Verification items for the finished model (mm, model axes). A direction names the side the tool comes from. Round coordinates to 2 decimals unless told otherwise and drop trailing zeros. Write each loop counter-clockwise with the first axis right and the second up, starting at its lowest first coordinate (ties: lowest second). Pieces come first, ordered by that corner, then holes. Notation, with made-up numbers: M -27.75,-32 L 7.25,-32 A15 ccw 7.25,-9 Z; hole C -29,80.25 d5. An arc over 180 degrees is marked long. Write each question's results on one line, items separated by ' | '.
from build123d import *

# Parameters (mm, degrees)
SKETCH2_W           = 21.826709
SKETCH2_H           = 6
SKETCH2_W_2         = 26.410128
SKETCH2_H_2         = 20
BOSS_EXTRUDE5_DEPTH = 0.7
BOSS_EXTRUDE6_DEPTH = 5
FILLET1_R           = 2.5


with BuildPart() as part:
    # Sketch2 → Boss-Extrude5 (new body)
    with BuildSketch(Plane.XY):
        Polygon((125.022768, -71), (125.022768, 0), (0, 0), (0, -71), (16.75, -71), align=None)
        with Locations((34.8557935, -61.193169)):
            Rectangle(SKETCH2_W, SKETCH2_H, mode=Mode.SUBTRACT)
        with Locations((55.882521, -16)):
            Rectangle(SKETCH2_W_2, SKETCH2_H_2, mode=Mode.SUBTRACT)
    extrude(amount=BOSS_EXTRUDE5_DEPTH)

    # Sketch2_9 → Boss-Extrude6 (add)
    with BuildSketch(Plane.XY):
        Polygon((9.375, -6.25), (18.625, -6.25), (14, -17.35), align=None)
        Polygon((17, -23.45), (23.75, -7.25), (23.75, -16.95), (17, -33.15), align=None)
        Polygon((11, -33.15), (11, -23.45), (4.25, -7.25), (4.25, -16.95), align=None)
        Polygon((107.138624, -23.45), (100.388624, -7.25), (100.388624, -16.95), (107.138624, -33.15), align=None)
        Polygon((105.513624, -6.25), (114.763624, -6.25), (110.138624, -17.35), align=None)
        Polygon((119.888624, -16.95), (113.138624, -33.15), (113.138624, -23.45), (119.888624, -7.25), align=None)
    extrude(amount=-BOSS_EXTRUDE6_DEPTH)

    # Fillet1
    fillet1_edges = [part.edges().sort_by_distance(p)[0] for p in [
        (23.942439, -64.193169, 0.35),
        (45.769148, -64.193169, 0.35),
        (45.769148, -58.193169, 0.35),
        (23.942439, -58.193169, 0.35),
        (42.677457, -26, 0.35),
        (69.087585, -26, 0.35),
        (69.087585, -6, 0.35),
        (42.677457, -6, 0.35),
    ]]
    fillet(fillet1_edges, radius=FILLET1_R)


solid = part.part
1) Sectioned sample at A-A, the plane x = 37. Record the cut outline in (y, z), and give its area (3 significant figures).
Calculated:
outline: M -71,0 L -64.19,0 L -64.19,0.7 L -71,0.7 Z; M -58.19,0 L 0,0 L 0,0.7 L -58.19,0.7 Z | area: 45.5 mm²
2) Sectioned sample at D-D, the plane y = -38.5. Record the cut outline in (x, z).
Calculated:
outline: M 0,0 L 125.02,0 L 125.02,0.7 L 0,0.7 Z
3) Material ranges on line 1 (X direction, y = -21, z = 0.2); line 2 (X direction, y = -13, z = -3.2); line 3 (X direction, y = -32, z = -0.5), recorded low to high. Write a range as [from, to].
Calculated:
line 1: x = [0, 42.68], [69.09, 125.02] | line 2: x = [4.25, 6.65], [12.19, 15.81], [21.35, 23.75], [100.39, 102.78], [108.33, 111.95], [117.49, 119.89] | line 3: x = [10.52, 11], [17, 17.48], [106.66, 107.14], [113.14, 113.62]
4) Access from +Z, -Z, +X, -X, +Y, -Y to the whole of each face (thin tool, end or side, straight path). Record for faces 1 (the flat face through (7.58, -24.94, -2.46)), 2 (the flat face through (116.56, -24.94, -2.46)), 3 (the flat face through (14, -6.25, -2)), 4 (the cylindrical face through (68.336, -25.287, 0.355)).
Calculated:
face 1: -Z, -X, -Y | face 2: -Z, +X, -Y | face 3: -Z, +X, -X, +Y | face 4: +Z, -Z
5) Sectioned sample at C-C, the plane x = 64. Record the cut outline in (y, z), and give its area (3 significant figures).
Calculated:
outline: M -71,0 L -26,0 L -26,0.7 L -71,0.7 Z; M -6,0 L 0,0 L 0,0.7 L -6,0.7 Z | area: 35.7 mm²
6) Sectioned sample at B-B, the plane z = -3.45. Record the cut outline in (x, y) (3 decimals), and give its area (3 significant figures).
Calculated:
outline: M 4.25,-16.95 L 11,-33.15 L 11,-23.45 L 4.25,-7.25 Z; M 9.375,-6.25 L 14,-17.35 L 18.625,-6.25 Z; M 17,-33.15 L 23.75,-16.95 L 23.75,-7.25 L 17,-23.45 Z; M 100.389,-16.95 L 107.139,-33.15 L 107.139,-23.45 L 100.389,-7.25 Z; M 105.514,-6.25 L 110.139,-17.35 L 114.764,-6.25 Z; M 113.139,-33.15 L 119.889,-16.95 L 119.889,-7.25 L 113.139,-23.45 Z | area: 365 mm²
7) Draft check along X on faces 5 (the flat face through (8, -20, -5)), 6 (the flat face through (119.889, -12, -2)), 7 (the cylindrical face through (68.375, -6.752, 0.355)). Enter one of: pulls with the +X half, pulls with the -X half, needs draft (parallel to the pull), parting line crosses it, or undercut.
Calculated:
face 5: needs draft | face 6: pulls with the +X half | face 7: undercut
8) Depth check by flat-ended pin: P1, Ø1.5, axis at y = -12, z = -3.5, coming from the -X side; P2, Ø2.5, axis at y = -12, z = -1.5, coming from the +X side; P3, Ø1, axis at x = 60, y = -53, coming from the -Z side. Enter the tip coordinate at first touch or a pass-through.
Calculated:
P1: stops at x = 4.25 | P2: stops at x = 119.89 | P3: stops at z = 0
